Design review of the part built by this model. Coordinates are the model's own, in mm. A direction names the side the tool comes from. Round coordinates to 2 decimals unless told otherwise and drop trailing zeros. Order: outer loops, then holes, each group sorted by start corner. A loop starts at its lowest first (then second) coordinate and runs counter-clockwise, first axis right, second up.
from build123d import *

# Parameters (mm, degrees)
SKETCH2_W          = 6.35
SKETCH2_H          = 6.35
CUT_EXTRUDE1_DEPTH = 195.31


with BuildPart() as part:
    # Sketch1 → Revolve1 (revolve)
    with BuildSketch(Plane(origin=(0, 0, 0), x_dir=(1, 0, 0), z_dir=(0, 1, 0))):
        Polygon((-106.68, 0), (106.68, 0), (106.68, 6.35), (87.63, 6.35), (87.63, 19.05), (-87.63, 19.05), (-87.63, 6.35), (-106.68, 6.35), align=None)
    revolve(axis=Axis((-106.68, 0, 0), (1, 0, 0)))

    # Sketch2 → Cut-Extrude1 (cut, through all)
    with BuildSketch(Plane(origin=(87.63, 0, 0), x_dir=(0, 0, -1), z_dir=(1, 0, 0))):
        with Locations((0, 15.875)):
            Rectangle(SKETCH2_W, SKETCH2_H)
        with Locations((0, -15.875)):
            Rectangle(SKETCH2_W, SKETCH2_H)
    extrude(amount=-CUT_EXTRUDE1_DEPTH, mode=Mode.SUBTRACT)


solid = part.part
1) The part is to be moulded in two halves that separate along Z. For faces 6 (the face through (-1.227, 0.374, 19.046)), 7 (the face through (-87.63, -8, 0)), 8 (the face through (1, -12.7, 0)), say which applies: released by +Z, released by -Z, zero draft, split by the parting line, or undercut.
Results:
face 6: released by +Z
face 7: zero draft
face 8: undercut
2) Take a section at A-A on z = 0. Give the boundary of the cut face in (x, y), plus the area to 3 significant figures.
Results:
outline: (-106.68, -6.35) - (-87.63, -6.35) - (-87.63, -12.7) - (87.63, -12.7) - (87.63, -6.35) - (106.68, -6.35) - (106.68, 6.35) - (87.63, 6.35) - (87.63, 12.7) - (-87.63, 12.7) - (-87.63, 6.35) - (-106.68, 6.35) - close
area: 4,940 mm2
3) To check wall thickness, follow line 1 along X through (y, z) = (-6.5, 14); line 2 along Z through (x, y) = (-25.5, 13) (3 decimals); line 3 along Z through (x, y) = (26, 3). State the ranges of each line that lie inside material, in increasing order.
Results:
line 1: x = -87.63 to 87.63
line 2: z = -13.925 to -3.175, 3.175 to 13.925
line 3: z = -18.81 to 18.81
4) Clearance check with flat-ended pins moving along their axes: P1, Ø1.8, axis at x = 2.5, y = -14.5, coming from the -Z side; P2, Ø3, axis at x = 30.5, z = 0, coming from the +Y side; P3, Ø3, axis at x = 33, y = 15, coming from the +Z side. State where each tip first meets the part, or that it passes through.
Results:
P1: stops at z = -13.34
P2: stops at y = 12.7
P3: stops at z = 13.44
5) Take a section at C-C on x = 40. Give the boundary of the cut face in (y, z) (3 decimals), plus the area to 3 significant figures.
Results:
outline: (-18.784, -3.175) arc R19.05 ccw to (18.784, -3.175) - (12.7, -3.175) - (12.7, 3.175) - (18.784, 3.175) arc R19.05 ccw to (-18.784, 3.175) - (-12.7, 3.175) - (-12.7, -3.175) - close
area: 1,060 mm2
6) For faces 1 (the face through (87.63, -8, 0)), 2 (the face through (1, 16, 3.175)), 3 (the face through (-97.29, -6.2, 1.38)), 4 (the face through (-1.227, -0.374, -19.046)), 5 (the face through (1, -16, 3.175)), list the 3-axis set-ups (+Z, -Z, +X, -X, +Y, -Y) from which the entire face can be reached by the end or side of a thin tool; tool diameter is ignored.
Results:
face 1: +X
face 2: +X, -X, +Y
face 3: -X
face 4: -Z, +X, -X
face 5: +X, -X, -Y
7) Take a section at B-B on y = 0. Give the boundary of the cut face in (x, z).
Results:
outline: (-106.68, -6.35) - (-87.63, -6.35) - (-87.63, -19.05) - (87.63, -19.05) - (87.63, -6.35) - (106.68, -6.35) - (106.68, 6.35) - (87.63, 6.35) - (87.63, 19.05) - (-87.63, 19.05) - (-87.63, 6.35) - (-106.68, 6.35) - close
8) Take a section at D-D on z = -10. Give the boundary of the cut face in (x, y), plus the area to 3 significant figures.
Results:
outline: (-87.63, -16.21) - (87.63, -16.21) - (87.63, 16.21) - (-87.63, 16.21) - close
area: 5,680 mm2
